Geometry check sheet. Reference: the model listing, model coordinates, mm. A direction names the side the tool comes from. Coordinates: 2 decimals unless noted, no trailing zeros. Write each loop counter-clockwise with the first axis right and the second up, starting at its lowest first coordinate (ties: lowest second). Pieces come first, ordered by that corner, then holes. Notation, with made-up numbers: (48, -35.5) -> (93, -35.5) arc R23 ccw to (93, -14.5) -> close; hole circle Ø3 at (40, 21.25). An arc over 180 degrees is marked (long way). Answer in a Markdown table with one row per item. Add a question column.
1. Cross-section at B-B on x = -1.75. Record the cut outline in (y, z).
2. Depth check by flat-ended pin: P1, Ø1.5, axis at y = -5.5, z = 2, coming from the -X side; P2, Ø1, axis at x = -10.5, z = 3.5, coming from the +Y side; P3, Ø2, axis at x = 6.5, z = 3, coming from the -Y side. Enter the tip coordinate at first touch or a pass-through.
3. Cross-section at C-C on z = 0.7. Record the cut outline in (x, y).
4. Scan lines: L1, parallel to Y at x = -0.5, z = 0.75; L2, parallel to Y at x = -1.5, z = 3.8; L3, parallel to X at y = 1.75, z = 3.8. Record each from-to range of solid material in increasing order. Write a range as from..to.
5. Mould release check, pull along X, two halves, no side actions. Record for faces 3 (the flat face through (-6, -3, 4.4)), 4 (the cylindrical face through (9.885, 5.288, 2.169)), 5 (the cylindrical face through (-11.983, -3.751, 2.169)): pulls with the +X half, pulls with the -X half, needs draft (parallel to the pull), parting line crosses it, or undercut.
6. Cross-section at A-A on y = 3.25. Record the cut outline in (x, z), and give its area (3 significant figures).
7. Cross-section at D-D on y = 9.75. Record the cut outline in (x, z).
8. Set-up check for faces 1 (the flat face through (-5.66, -3.2, 2.17)), 2 (the cylindrical face through (-0.363, -11.204, 2.169)): record each of +Z, -Z, +X, -X, +Y, -Y from which the full face is reachable in a straight line by a thin tool's end or side.
```python
from build123d import *

# Parameters (mm, degrees)
BOSS_EXTRUDE1_DEPTH = 4.4


with BuildPart() as part:
    # Sketch1 → Boss-Extrude1 (new body)
    with BuildSketch(Plane.XY):
        with BuildLine():
            ThreePointArc((-7.106112246, 6.995417074), (2.908276026, 12.245932527), (12.355783111, 6.033002876))
            ThreePointArc((12.355783111, 6.033002876), (9.860301204, 5.257635244), (9.611265019, 2.65636519))
            ThreePointArc((9.611265019, 2.65636519), (9.151150649, -8.641607183), (-0.953157804, -13.716923496))
            ThreePointArc((-0.953157804, -13.716923496), (-0.376904917, -11.168088953), (-2.505152773, -9.651782264))
            ThreePointArc((-2.505152773, -9.651782264), (-12.059426674, -3.604325344), (-11.402625308, 7.68392062))
            ThreePointArc((-11.402625308, 7.68392062), (-9.483396287, 5.910453709), (-7.106112246, 6.995417074))
        make_face()
        Polygon((7.505553499, 0), (3.75277675, 6.5), (-3.75277675, 6.5), (-7.505553499, 0), (-3.75277675, -6.5), (3.75277675, -6.5), align=None, mode=Mode.SUBTRACT)
    extrude(amount=BOSS_EXTRUDE1_DEPTH)


solid = part.part
```
Results found:
| question | item | result |
|---|---|---|
| 1 | outline | (-9.8, 0) -> (-6.5, 0) -> (-6.5, 4.4) -> (-9.8, 4.4) -> close; (6.5, 0) -> (11.47, 0) -> (11.47, 4.4) -> (6.5, 4.4) -> close |
| 2 | P1 | stops at x = -11.38 |
| 2 | P2 | stops at y = 6.83 |
| 2 | P3 | stops at y = -12.17 |
| 3 | outline | (-11.4, 7.68) arc R11.14 ccw to (-2.51, -9.65) arc R2.36 cw to (-0.95, -13.72) arc R11.14 ccw to (9.61, 2.66) arc R2.36 cw to (12.36, 6.03) arc R11.14 ccw to (-7.11, 7) arc R2.36 cw to start; hole (-7.51, 0) -> (-3.75, -6.5) -> (3.75, -6.5) -> (7.51, 0) -> (3.75, 6.5) -> (-3.75, 6.5) -> close |
| 4 | L1 | y = -13.74..-13.12, -10.9..-6.5, 6.5..11.89 |
| 4 | L2 | y = -9.91..-6.5, 6.5..11.57 |
| 4 | L3 | x = -13.29..-6.5, 6.5..10.05 |
| 5 | face 3 | needs draft |
| 5 | face 4 | undercut |
| 5 | face 5 | pulls with the -X half |
| 6 | outline | (-13.15, 0) -> (-5.63, 0) -> (-5.63, 4.4) -> (-13.15, 4.4) -> close; (5.63, 0) -> (9.39, 0) -> (9.39, 4.4) -> (5.63, 4.4) -> close |
| 6 | area | 49.6 mm^2 |
| 7 | outline | (-4.69, 0) -> (9.4, 0) -> (9.4, 4.4) -> (-4.69, 4.4) -> close |
| 8 | face 1 | +Z, -Z |
| 8 | face 2 | +Z, -Z, -X |
